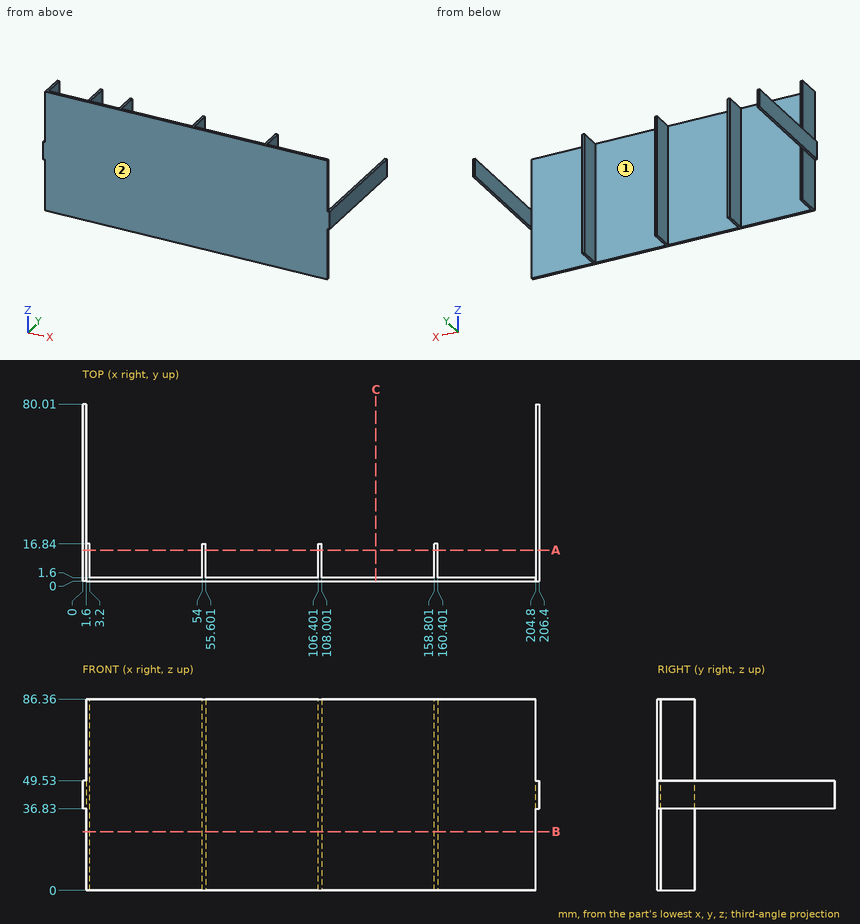
Geometry check sheet. Reference: drawing and pictorial views, mm from the part's lowest x, y, z. A direction names the side the tool comes from. Coordinates: 2 decimals unless noted, no trailing zeros. Order: outer loops, then holes, each group sorted by start corner. A loop starts at its lowest first (then second) coordinate and runs counter-clockwise, first axis right, second up. Notation, with made-up numbers: (29.5, -20.75) -> (54.5, -20.75) arc R34 cw to (54.5, 18.25) -> close; hole circle Ø2 at (17.25, 31.25). An arc over 180 degrees is marked (long way). Write item = value, one per line. Start each with the question number.
1) Cross-section at C-C (x = 132.5). Enter the section's corners in (y, z), then the cut area to 3 significant figures.
2) Cross-section at B-B (z = 26.5). Enter the section's corners in (x, y).
3) Material ranges on L1, parallel to X at y = 14.5, z = 25.5; L2, parallel to X at y = 34, z = 47.5; L3, parallel to X at y = 13, z = 43, recorded low to high.
4) Access from +Z, -Z, +X, -X, +Y, -Y to the whole of each face (thin tool, end or side, straight path). Record for the marked faces 1 and 2.
5) Go/stop test with flat-tipped pins: P1, Ø7.5, axis at y = 9.5, z = 25, coming from the -X side; P2, Ø4, axis at x = 156.5, z = 21, coming from the +Y side; P3, Ø1.8, axis at x = 0.5, y = 31.5, coming from the -Z side; P4, Ø6, axis at x = 157, y = 20, coming from the -Z side. Record where each tip stops, or that it passes through.
6) Cross-section at A-A (y = 14). Enter the section's corners in (x, z).
Ans:
q1.outline = (0, 0) -> (1.6, 0) -> (1.6, 86.36) -> (0, 86.36) -> close
q1.area = 138 mm²
q2.outline = (1.6, 0) -> (204.8, 0) -> (204.8, 1.6) -> (160.4, 1.6) -> (160.4, 16.84) -> (158.8, 16.84) -> (158.8, 1.6) -> (108, 1.6) -> (108, 16.84) -> (106.4, 16.84) -> (106.4, 1.6) -> (55.6, 1.6) -> (55.6, 16.84) -> (54, 16.84) -> (54, 1.6) -> (3.2, 1.6) -> (3.2, 16.84) -> (1.6, 16.84) -> close
q3.L1 = 1.6 to 3.2, 54 to 55.6, 106.4 to 108, 158.8 to 160.4
q3.L2 = 0 to 1.6, 204.8 to 206.4
q3.L3 = 0 to 3.2, 54 to 55.6, 106.4 to 108, 158.8 to 160.4, 204.8 to 206.4
q4.face_1 = +Z, -Z, +Y
q4.face_2 = +Z, -Z, +X, -X, -Y
q5.P1 = 1.6
q5.P2 = 1.6
q5.P3 = 36.83
q5.P4 = through
q6.outline = (0, 36.83) -> (1.6, 36.83) -> (1.6, 0) -> (3.2, 0) -> (3.2, 86.36) -> (1.6, 86.36) -> (1.6, 49.53) -> (0, 49.53) -> close; (54, 0) -> (55.6, 0) -> (55.6, 86.36) -> (54, 86.36) -> close; (106.4, 0) -> (108, 0) -> (108, 86.36) -> (106.4, 86.36) -> close; (158.8, 0) -> (160.4, 0) -> (160.4, 86.36) -> (158.8, 86.36) -> close; (204.8, 36.83) -> (206.4, 36.83) -> (206.4, 49.53) -> (204.8, 49.53) -> close
